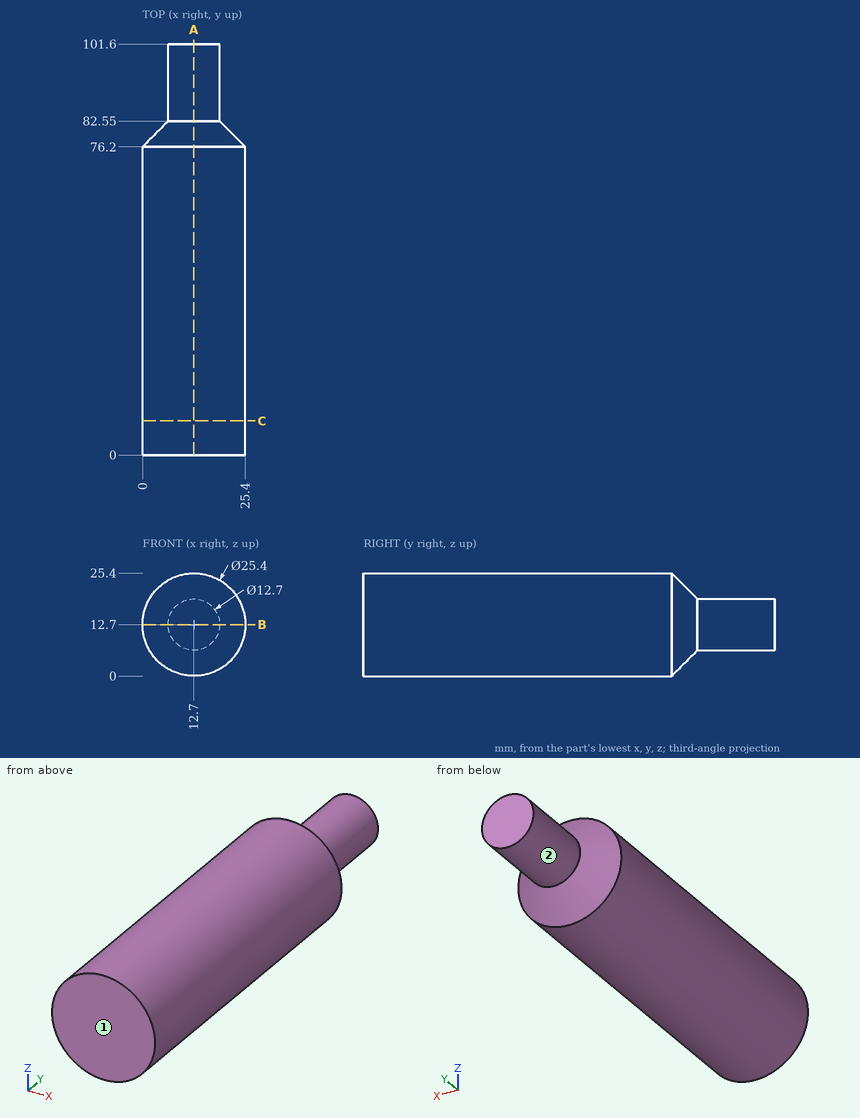
Check sheet for the drawn part. Datum: minimum x, y, z corner. Units: mm. A direction names the side the tool comes from. Give positions to 0.01 mm unless a question says otherwise; leave off trailing zeros. Write each loop counter-clockwise with the first axis right and the second up, starting at its lowest first coordinate (ties: lowest second). Pieces come first, ordered by that corner, then holes.
(1) Gauge pin test, flat ends, axial feed: pin 1 (3 mm diameter, centred on y = 90, z = 13.5, fed in from +X); pin 2 (4 mm diameter, centred on x = 17.5, y = 27, fed in from +Z); pin 3 (10 mm diameter, centred on x = 4.5, y = 83.5, fed in from +Z). Record the tip position at first contact, or that the pin passes through.
(2) Cross-section at C-C (y = 8.5). Enter the section's corners in (x, z), plus the area to 3 significant figures.
(3) Cross-section at B-B (z = 12.7). Enter the section's corners in (x, y).
(4) Access from +Z, -Z, +X, -X, +Y, -Y to the whole of each face (thin tool, end or side, straight path). Record for the marked faces 1 and 2.
(5) Cross-section at A-A (x = 12.7). Enter the section's corners in (y, z), plus the area to 3 significant figures.
(6) Material ranges on line 1 (Z direction, x = 13, y = 97.5); line 2 (Z direction, x = 13.25, y = 37.5); line 3 (Y direction, x = 18.75, z = 15.25), recorded low to high.
Worked out:
1. pin 1: stops at x = 19.05
1. pin 2: stops at z = 25.09
1. pin 3: stops at z = 20.59
2. outline: circle Ø25.4 at (12.7, 12.7)
2. area: 507 mm2
3. outline: (0, 0) - (25.4, 0) - (25.4, 76.2) - (19.05, 82.55) - (19.05, 101.6) - (6.35, 101.6) - (6.35, 82.55) - (0, 76.2) - close
4. face 1: +Z, -Z, +X, -X, -Y
4. face 2: +Y
5. outline: (0, 0) - (76.2, 0) - (82.55, 6.35) - (101.6, 6.35) - (101.6, 19.05) - (82.55, 19.05) - (76.2, 25.4) - (0, 25.4) - close
5. area: 2,300 mm2
6. line 1: z = 6.36 to 19.04
6. line 2: z = 0.01 to 25.39
6. line 3: y = 0 to 82.33
